from build123d import *

# Parameters (mm, degrees)
SKETCH_1_W          = 22
SKETCH_1_H          = 15
EXTRUDE_1_DEPTH     = 2.3
SKETCH_2_W          = 18.7
SKETCH_2_H          = 13.7
EXTRUDE_2_DEPTH     = 12.4
SKETCH_3_W          = 13.7
SKETCH_3_H          = 1.5
EXTRUDE_3_DEPTH     = 1.65
SKETCH_4_W          = 13.7
SKETCH_4_H          = 1.5
EXTRUDE_4_DEPTH     = 1.65
CUT_EXTRUDE_1_DEPTH = 10
SKETCH_5_R          = 1.18
EXTRUDE_5_DEPTH     = 9.5
FILLET_6_R          = 1


with BuildPart() as part:
    # 草图1 → 凸台-拉伸1 (new body)
    with BuildSketch(Plane(origin=(0, 0, 0), x_dir=(1, 0, 0), z_dir=(0, 1, 0))):
        Rectangle(SKETCH_1_W, SKETCH_1_H)
    extrude(amount=EXTRUDE_1_DEPTH)

    # 草图2 → 凸台-拉伸2 (add)
    with BuildSketch(Plane.XZ):
        with Locations((0, -0.65)):
            Rectangle(SKETCH_2_W, SKETCH_2_H)
    extrude(amount=EXTRUDE_2_DEPTH)

    # 草图3 → 凸台-拉伸3 (add)
    with BuildSketch(Plane.ZY.offset(9.35)):
        with Locations((-0.65, -2.55)):
            Rectangle(SKETCH_3_W, SKETCH_3_H)
    extrude(amount=EXTRUDE_3_DEPTH)

    # 草图4 → 凸台-拉伸4 (add)
    with BuildSketch(Plane(origin=(9.35, 0, 0), x_dir=(0, 0, -1), z_dir=(1, 0, 0))):
        with Locations((0.65, -2.55)):
            Rectangle(SKETCH_4_W, SKETCH_4_H)
    extrude(amount=EXTRUDE_4_DEPTH)

    # 草图6 → 切除-拉伸1 (cut)
    with BuildSketch(Plane(origin=(0, 2.3, 0), x_dir=(1, 0, 0), z_dir=(0, 1, 0))):
        with BuildLine():
            Line((0.405473154, -2.237773908), (1.757477388, -4.1))
            Line((1.757477388, -4.1), (4.3, -4.1))
            ThreePointArc((4.3, -4.1), (8.4, 0), (4.3, 4.1))
            Line((4.3, 4.1), (1.757477388, 4.1))
            Line((1.757477388, 4.1), (0.405473154, 2.237773908))
            ThreePointArc((0.405473154, 2.237773908), (0.000356772, 2.031527095), (-0.404340983, 2.238594131))
            Line((-0.404340983, 2.238594131), (-1.75, 4.1))
            Line((-1.75, 4.1), (-4.3, 4.1))
            ThreePointArc((-4.3, 4.1), (-8.4, 0), (-4.3, -4.1))
            Line((-4.3, -4.1), (-1.75, -4.1))
            Line((-1.75, -4.1), (-0.404340983, -2.238594131))
            ThreePointArc((-0.404340983, -2.238594131), (0.000356772, -2.031527095), (0.405473154, -2.237773908))
        make_face()
    extrude(amount=-CUT_EXTRUDE_1_DEPTH, mode=Mode.SUBTRACT)

    # 草图5 → 凸台-拉伸5 (add)
    with BuildSketch(Plane(origin=(0, -7.7, 0), x_dir=(1, 0, 0), z_dir=(0, 1, 0))):
        with Locations((-4.3, 0)):
            Circle(SKETCH_5_R)
        with Locations((4.3, 0)):
            Circle(SKETCH_5_R)
    extrude(amount=EXTRUDE_5_DEPTH)

    # 圆角6
    fillet_6_edges = [part.edges().sort_by_distance(p)[0] for p in [
        (-5.48, 1.8, 0),
        (3.12, 1.8, 0),
    ]]
    fillet(fillet_6_edges, radius=FILLET_6_R)


solid = part.part
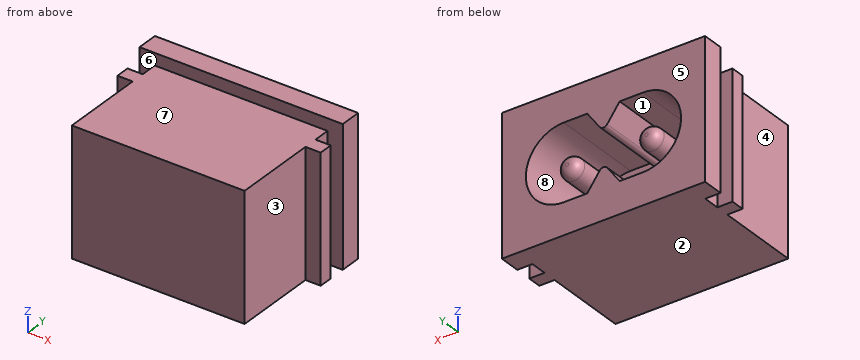
For this review, take the finished solid that the model builds, in its own axes (mm). Face numbers are marked on the shaded views. A direction names the side the tool comes from. Coordinates: 2 decimals unless noted, no trailing zeros. Write each loop counter-clockwise with the first axis right and the second up, starting at its lowest first coordinate (ties: lowest second). Pieces come first, ordered by that corner, then holes. Notation, with made-up numbers: (-13.5, 5.25) -> (27.5, 5.25) arc R6 cw to (27.5, 16.25) -> close; hole circle Ø10 at (20, -29.5). An arc over 180 degrees is marked (long way). Write each question's results on one line, items separated by ' | '. Start each with the question number.
1) The part is to be moulded in two halves that separate along X. For the marked faces 1, 2 and 3, say which applies: +X half, -X half, draft (parallel to the pull), parting line (faces both ways), or undercut.
2) Wall thickness on L1, parallel to Z at x = 2, y = -6; L2, parallel to X at y = -5.5, z = 3.5; L3, parallel to Z at x = 0, y = -7: over which ranges is each line inside the solid? List them lowest first. Write a range as [from, to].
3) Consider section A-A (y = -1). Write out the cut boundary in (x, z), plus the area to 3 significant figures.
4) For the marked faces 4, 5, 6, 7 and 8, list the 3-axis set-ups (+Z, -Z, +X, -X, +Y, -Y) from which the entire face can be reached by the end or side of a thin tool; tool diameter is ignored.
5) Consider section C-C (x = 7.25). Write out the cut boundary in (y, z), plus the area to 3 significant figures.
6) Consider section B-B (z = -5.75). Write out the cut boundary in (x, y), plus the area to 3 significant figures.
7) Consider section D-D (z = -3). Write out the cut boundary in (x, y), plus the area to 3 significant figures.
8) Insertion check: pin 1 (1 mm diameter, centred on x = -1.5, z = 0.5, fed in from +Y); pin 2 (0.5 mm diameter, centred on x = -10.5, z = -1, fed in from -Y); pin 3 (2 mm diameter, centred on y = -7.5, z = -3.5, fed in from +X). Each pin has a flat end and moves straight along its axis. Give the tip position at first contact, or say it passes through.
Geometry says:
1) face 1: undercut | face 2: draft | face 3: +X half
2) L1: [-7.5, -4.1], [4.1, 6.2] | L2: [-9.35, -6.44], [-1.32, 1.32], [6.44, 9.35] | L3: [-7.5, -2.03], [2.03, 6.2]
3) outline: (-9.35, -7.5) -> (9.35, -7.5) -> (9.35, 6.2) -> (-9.35, 6.2) -> close; circle Ø2.36 at (-4.3, 0); circle Ø2.36 at (4.3, 0); hole (-4.3, -4.1) -> (-1.75, -4.1) -> (-0.4, -2.24) arc R0.5 cw to (0.41, -2.24) -> (1.76, -4.1) -> (4.3, -4.1) arc R4.1 ccw to (4.3, 4.1) -> (1.76, 4.1) -> (0.41, 2.24) arc R0.5 cw to (-0.4, 2.24) -> (-1.75, 4.1) -> (-4.3, 4.1) arc R4.1 ccw to start | area: 150 mm^2
4) face 4: +Z, -Z, -X, -Y | face 5: +Z, -Z, +X, -X, +Y | face 6: +Z | face 7: +Z, +X, -X, -Y | face 8: +Y
5) outline: (-12.4, -7.5) -> (2.3, -7.5) -> (2.3, -2.85) -> (-7.7, -2.85) -> (-7.7, 2.85) -> (2.3, 2.85) -> (2.3, 7.5) -> (0, 7.5) -> (0, 6.2) -> (-12.4, 6.2) -> close | area: 147 mm^2
6) outline: (-11, -3.3) -> (-9.35, -3.3) -> (-9.35, -12.4) -> (9.35, -12.4) -> (9.35, -3.3) -> (11, -3.3) -> (11, -1.8) -> (9.35, -1.8) -> (9.35, 0) -> (11, 0) -> (11, 2.3) -> (-11, 2.3) -> (-11, 0) -> (-9.35, 0) -> (-9.35, -1.8) -> (-11, -1.8) -> close | area: 287 mm^2
7) outline: (-11, -3.3) -> (-9.35, -3.3) -> (-9.35, -12.4) -> (9.35, -12.4) -> (9.35, -3.3) -> (11, -3.3) -> (11, -1.8) -> (9.35, -1.8) -> (9.35, 0) -> (11, 0) -> (11, 2.3) -> (7.09, 2.3) -> (7.09, -7.7) -> (0.96, -7.7) -> (0.96, 2.3) -> (-0.95, 2.3) -> (-0.95, -7.7) -> (-7.09, -7.7) -> (-7.09, 2.3) -> (-11, 2.3) -> (-11, 0) -> (-9.35, 0) -> (-9.35, -1.8) -> (-11, -1.8) -> close | area: 165 mm^2
8) pin 1: y = -7.7 | pin 2: y = -3.3 | pin 3: x = 9.35
